```python
from build123d import *

# Parameters (mm, degrees)
BOSS_EXTRUDE1_DEPTH = 0.7


with BuildPart() as part:
    # Sketch1 → Boss-Extrude1 (new body)
    with BuildSketch(Plane.XY):
        with BuildLine():
            Line((-2.561408424, -2.557883579), (-1.879385242, -0.684040287))
            ThreePointArc((-1.879385242, -0.684040287), (-1.99891759, -0.065791087), (-1.920297211, 0.558979983))
            ThreePointArc((-1.920297211, 0.558979983), (-1.937015688, 0.781382977), (-2.095699977, 0.938105328))
            Line((-2.095699977, 0.938105328), (-2.701605558, 1.209328909))
            ThreePointArc((-2.701605558, 1.209328909), (-2.995016962, 1.548683887), (-2.923070831, 1.991488368))
            ThreePointArc((-2.923070831, 1.991488368), (-2.122951492, 2.829036225), (-1.095155737, 3.363183449))
            ThreePointArc((-1.095155737, 3.363183449), (-0.649889409, 3.308503006), (-0.406063751, 2.931938136))
            Line((-0.406063751, 2.931938136), (-0.314993353, 2.274374461))
            ThreePointArc((-0.314993353, 2.274374461), (0, 2), (0.314993353, 2.274374461))
            Line((0.314993353, 2.274374461), (0.406063751, 2.931938136))
            ThreePointArc((0.406063751, 2.931938136), (0.649889409, 3.308503006), (1.095155737, 3.363183449))
            ThreePointArc((1.095155737, 3.363183449), (2.122951492, 2.829036225), (2.923070831, 1.991488368))
            ThreePointArc((2.923070831, 1.991488368), (2.995016962, 1.548683887), (2.701605558, 1.209328909))
            Line((2.701605558, 1.209328909), (2.095699977, 0.938105328))
            ThreePointArc((2.095699977, 0.938105328), (1.937015688, 0.781382977), (1.920297211, 0.558979983))
            ThreePointArc((1.920297211, 0.558979983), (1.99891759, -0.065791087), (1.879385242, -0.684040287))
            Line((1.879385242, -0.684040287), (2.561408424, -2.557883579))
            ThreePointArc((2.561408424, -2.557883579), (3.113603209, -3.004615598), (3.76702433, -2.726174553))
            ThreePointArc((3.76702433, -2.726174553), (0, 4.65), (-3.76702433, -2.726174553))
            ThreePointArc((-3.76702433, -2.726174553), (-3.113603209, -3.004615598), (-2.561408424, -2.557883579))
        make_face()
    extrude(amount=-BOSS_EXTRUDE1_DEPTH)


solid = part.part
```
Can you work these out from the model? Positions are in its coordinate system, mm. A direction names the side the tool comes from. Coordinates: 2 decimals unless noted, no trailing zeros. Loops run counter-clockwise (first coordinate to the right, second up) from the corner with the lowest first, then second, coordinate; pieces in that order, holes last.
Item 1: I'm going to push a flat-ended pin straight in: pin 1 (1.5 mm diameter, centred on x = 1, y = 2.5, fed in from -Z). Where does the tip first touch, or does it pass through?
Answers below:
pin 1: stops at z = -0.7
Item 2: Which directions (+Z, -Z, +X, -X, +Y, -Y) give clear straight access to the entire face, cutting with the end or side of a thin tool? Please do faces 1 (the face through (2.11, 2.84, -0.35)), 2 (the face through (0, 3, 0)).
Answers below:
face 1: +Z, -Z
face 2: +Z, +X, -X, +Y, -Y
Item 3: Please list where these lines run through material, in increasing order: L1, parallel to X at y = 3, z = -0.3; L2, parallel to X at y = 2.25, z = -0.6; L3, parallel to X at y = 1.5, z = -0.2.
Answers below:
L1: x = -3.55 to -1.87, -0.42 to 0.42, 1.87 to 3.55
L2: x = -4.07 to -2.73, -0.31 to 0.31, 2.73 to 4.07
L3: x = -4.4 to -2.98, 2.98 to 4.4
Item 4: Suppose I cut it at C-C (y = 1.75). Please give me the cut outline in (x, z).
Answers below:
outline: (-4.31, -0.7) - (-3.01, -0.7) - (-3.01, 0) - (-4.31, 0) - close; (3.01, -0.7) - (4.31, -0.7) - (4.31, 0) - (3.01, 0) - close
Item 5: If we mould it in two halves opening along X, with no side actions, what happens to faces 3 (the face through (0, 3, -0.7)), 4 (the face through (-2.136, 2.819, -0.345)), 5 (the face through (0.143, 4.648, -0.345))? For each: released by +X, released by -X, zero draft, split by the parting line, or undercut.
Answers below:
face 3: zero draft
face 4: undercut
face 5: split by the parting line
Item 6: Suppose I cut it at D-D (x = 0). Please give me the cut outline in (y, z), then the cut area to 4 significant figures.
Answers below:
outline: (2, -0.7) - (4.65, -0.7) - (4.65, 0) - (2, 0) - close
area: 1.855 mm2
Item 7: Suppose I cut it at B-B (z = -0.1). Please give me the cut outline in (x, y) (3 decimals), then the cut area to 3 significant figures.
Answers below:
outline: (-3.767, -2.726) arc R0.689 ccw to (-2.561, -2.558) - (-1.879, -0.684) arc R2 cw to (-1.92, 0.559) arc R0.318 ccw to (-2.096, 0.938) - (-2.702, 1.209) arc R0.53 cw to (-2.923, 1.991) arc R3.537 cw to (-1.095, 3.363) arc R0.53 cw to (-0.406, 2.932) - (-0.315, 2.274) arc R0.318 ccw to (0.315, 2.274) - (0.406, 2.932) arc R0.53 cw to (1.095, 3.363) arc R3.537 cw to (2.923, 1.991) arc R0.53 cw to (2.702, 1.209) - (2.096, 0.938) arc R0.318 ccw to (1.92, 0.559) arc R2 cw to (1.879, -0.684) - (2.561, -2.558) arc R0.689 ccw to (3.767, -2.726) arc R4.65 ccw (long way) to start
area: 31.7 mm2
Item 8: Suppose I cut it at A-A (y = 0). Please give me the cut outline in (x, z).
Answers below:
outline: (-4.65, -0.7) - (-2, -0.7) - (-2, 0) - (-4.65, 0) - close; (2, -0.7) - (4.65, -0.7) - (4.65, 0) - (2, 0) - close
